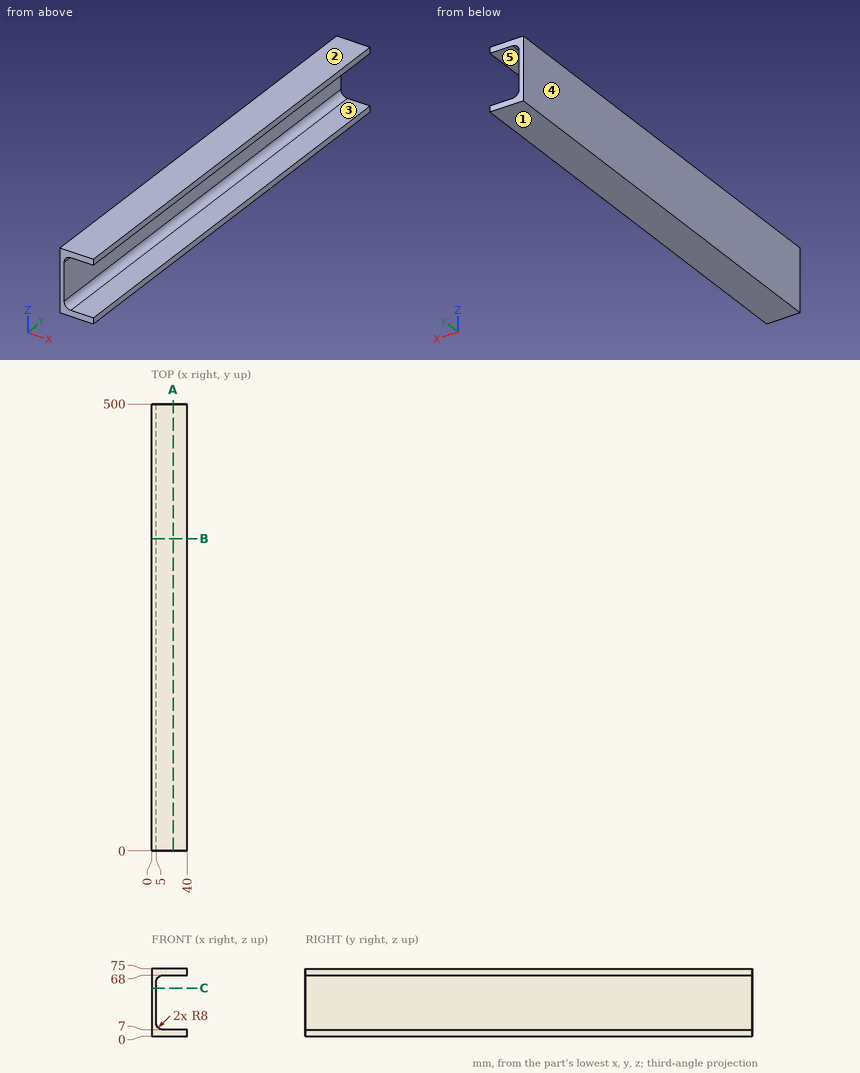
Geometry check sheet. Reference: drawing and pictorial views, mm from the part's lowest x, y, z. A direction names the side the tool comes from. Coordinates: 2 decimals unless noted, no trailing zeros. Order: outer loops, then holes, each group sorted by start corner. A loop starts at its lowest first (then second) coordinate and runs counter-clockwise, first axis right, second up.
Item 1: Section check A-A (x = 24). Enter the section's corners in (y, z).
Item 2: Mould release check, pull along Z, two halves, no side actions. Record for the marked faces 1, 2 and 3: released by +Z, released by -Z, zero draft, split by the parting line, or undercut.
Item 3: Section check C-C (z = 53.5). Enter the section's corners in (x, y), plus the area to 3 significant figures.
Item 4: Tool access check on the marked faces 4 and 5. Record the directions out of +Z, -Z, +X, -X, +Y, -Y that give a thin tool (end or side, any length) a straight path to the whole face; none if there is none.
Item 5: Scan lines: line 1 along Z through (x, y) = (16.5, 138.5); line 2 along X through (y, z) = (229, 39); line 3 along X through (y, z) = (201.5, 61). Record each from-to range of solid material in increasing order.
Item 6: Depth check by flat-ended pin: pin 1 (12 mm diameter, centred on y = 63, z = 9.5, fed in from +X); pin 2 (1 mm diameter, centred on y = 248, z = 50, fed in from +X). Enter the tip coordinate at first touch or a pass-through.
Item 7: Section check B-B (y = 349.5). Enter the section's corners in (x, z).
Check sheet entries:
1. outline: (0, 0) - (500, 0) - (500, 7) - (0, 7) - close; (0, 68) - (500, 68) - (500, 75) - (0, 75) - close
2. face 1: released by -Z
2. face 2: released by +Z
2. face 3: undercut
3. outline: (0, 0) - (5, 0) - (5, 500) - (0, 500) - close
3. area: 2,500 mm2
4. face 4: +Z, -Z, -X, +Y, -Y
4. face 5: +X, +Y, -Y
5. line 1: z = 0 to 7, 68 to 75
5. line 2: x = 0 to 5
5. line 3: x = 0 to 5.06
6. pin 1: stops at x = 40
6. pin 2: stops at x = 5
7. outline: (0, 0) - (40, 0) - (40, 7) - (13, 7) arc R8 cw to (5, 15) - (5, 60) arc R8 cw to (13, 68) - (40, 68) - (40, 75) - (0, 75) - close
